Design review of the part built by this model. Coordinates are the model's own, in mm. A direction names the side the tool comes from. Coordinates: 2 decimals unless noted, no trailing zeros. Loops run counter-clockwise (first coordinate to the right, second up) from the corner with the lowest first, then second, coordinate; pieces in that order, holes last. Notation, with made-up numbers: (84.25, 22) - (95.25, 22) arc R28 ccw to (95.25, 46) - close; hole circle Ø10 at (66, 22.5). An arc over 180 degrees is marked (long way). Answer in a Markdown table with one row per item. Add a question column.
(1) For faces 1 (the face through (9.1, 34.14, -29.9)), 2 (the face through (9.1, -34.14, -29.9)), 3 (the face through (-18, 0, -20)), 4 (the face through (-2.17, -9.76, 11.13)), 5 (the face through (17, 0, -20)), list the 3-axis set-ups (+Z, -Z, +X, -X, +Y, -Y) from which the entire face can be reached by the end or side of a thin tool; tool diameter is ignored.
(2) We need section C-C, the plane x = -15. Write out the cut boundary in (y, z).
(3) Clearance check with flat-ended pins moving along their axes: pin 1 (8 mm diameter, centred on x = 8, z = -26, fed in from -Y); pin 2 (1.5 mm diameter, centred on x = 12, y = -26, fed in from -Z); pin 3 (2.5 mm diameter, centred on x = 15.5, y = 4.5, fed in from -Z); pin 4 (8 mm diameter, centred on x = -14.5, y = 25.5, fed in from +Z). State where each tip first meets the part, or that it passes through.
(4) We need section D-D, the plane y = 20.5. Write out the cut boundary in (x, z), plus the area to 3 significant figures.
(5) We need section A-A, the plane y = 0. Write out the cut boundary in (x, z).
(6) To check wall thickness, follow L1, parallel to Z at x = -13, y = -5; L2, parallel to Z at x = 0, y = 17.5; L3, parallel to X at y = -2.5, z = -34.5. State the ranges of each line that lie inside material, in increasing order. Write a range as [from, to].
(7) We need section B-B, the plane z = -34.5. Write out the cut boundary in (x, y).
from build123d import *

# Parameters (mm, degrees)
BOSS_EXTRUDE1_DEPTH = 35
SKETCH2_R           = 10
BOSS_EXTRUDE2_DEPTH = 20
FILLET1_R           = 3
CHAMFER1_SIZE       = 0.5


with BuildPart() as part:
    # Sketch1 → Boss-Extrude1 (new, symmetric)
    with BuildSketch(Plane(origin=(0, 0, 0), x_dir=(1, 0, 0), z_dir=(0, 1, 0))):
        Polygon((25, 0), (-25, 0), (-25, 20), (-10, 20), (-10, 40), (10, 40), (10, 20), (25, 20), align=None)
    extrude(amount=BOSS_EXTRUDE1_DEPTH, both=True)

    # Sketch2 → Boss-Extrude2 (add)
    with BuildSketch(Plane.XY):
        Circle(SKETCH2_R)
    extrude(amount=BOSS_EXTRUDE2_DEPTH)

    # Fillet1
    fillet1_edges = [part.edges().sort_by_distance(p)[0] for p in [
        (25, -35, -10),
        (0, -35, 0),
        (-25, -35, -10),
        (-17.5, -35, -20),
        (0, 35, 0),
        (-10, 0, -20),
        (-10, 0, -40),
        (10, 0, -40),
        (10, 0, -20),
        (25, 0, -20),
        (25, 0, 0),
        (-25, 0, 0),
        (-25, 0, -20),
        (25, 35, -10),
        (17.5, 35, -20),
        (-10, 0, 0),
        (10, 35, -30),
        (0, 35, -40),
        (-10, 35, -30),
        (-17.5, 35, -20),
        (-10, -35, -30),
        (-25, 35, -10),
        (0, -35, -40),
        (10, -35, -30),
        (17.5, -35, -20),
    ]]
    fillet(fillet1_edges, radius=FILLET1_R)

    # Chamfer1
    chamfer1_edges = [part.edges().sort_by_distance(p)[0] for p in [
        (-10, 0, 20),
    ]]
    chamfer(chamfer1_edges, length=CHAMFER1_SIZE)


solid = part.part
Responses:
| question | item | result |
|---|---|---|
| 1 | face 1 | -Z, +X, +Y |
| 1 | face 2 | -Z, +X, -Y |
| 1 | face 3 | -Z, -X, +Y, -Y |
| 1 | face 4 | +Z |
| 1 | face 5 | -Z, +X, +Y, -Y |
| 2 | outline | (-35, -17) arc R3 ccw to (-32, -20) - (32, -20) arc R3 ccw to (35, -17) - (35, -3) arc R3 ccw to (32, 0) - (-32, 0) arc R3 ccw to (-35, -3) - close |
| 3 | pin 1 | stops at y = -35 |
| 3 | pin 2 | stops at z = -20.56 |
| 3 | pin 3 | stops at z = -20 |
| 3 | pin 4 | stops at z = 0 |
| 4 | outline | (-25, -17) arc R3 ccw to (-22, -20) - (-13, -20) arc R3 cw to (-10, -23) - (-10, -37) arc R3 ccw to (-7, -40) - (7, -40) arc R3 ccw to (10, -37) - (10, -23) arc R3 cw to (13, -20) - (22, -20) arc R3 ccw to (25, -17) - (25, -3) arc R3 ccw to (22, 0) - (-22, 0) arc R3 ccw to (-25, -3) - close |
| 4 | area | 1,390 mm2 |
| 5 | outline | (-25, -17) arc R3 ccw to (-22, -20) - (-13, -20) arc R3 cw to (-10, -23) - (-10, -37) arc R3 ccw to (-7, -40) - (7, -40) arc R3 ccw to (10, -37) - (10, -23) arc R3 cw to (13, -20) - (22, -20) arc R3 ccw to (25, -17) - (25, -3) arc R3 ccw to (22, 0) - (13, 0) arc R3 cw to (10, 3) - (10, 19.5) - (9.5, 20) - (-9.5, 20) - (-10, 19.5) - (-10, 3) arc R3 cw to (-13, 0) - (-22, 0) arc R3 ccw to (-25, -3) - close |
| 6 | L1 | z = [-20, 0] |
| 6 | L2 | z = [-40, 0] |
| 6 | L3 | x = [-10, 10] |
| 7 | outline | (-10, -32) arc R3 ccw to (-7, -35) - (7, -35) arc R3 ccw to (10, -32) - (10, 32) arc R3 ccw to (7, 35) - (-7, 35) arc R3 ccw to (-10, 32) - close |
